```python
from build123d import *

# Parameters (mm, degrees)
BOSS_EXTRU_1_DEPTH       = 20
ESQUISSE2_W              = 10
ESQUISSE2_H              = 21
ENL_V_MAT_EXTRU_1_DEPTH  = 2.5
ESQUISSE3_R              = 1.5
ENL_V_MAT_EXTRU_2_DEPTH  = 20.384776311
ESQUISSE4_R              = 4.1
ENL_V_MAT_EXTRU_3_DEPTH  = 16.384776311
ESQUISSE5_R              = 1.25
ENL_V_MAT_EXTRU_4_DEPTH  = 17.207106781
BOSS_EXTRU_2_DEPTH       = 1
ENL_V_MAT_EXTRU_7_DEPTH  = 11
ENL_V_MAT_EXTRU_8_DEPTH  = 11
ESQUISSE11_R             = 1.5
ENL_V_MAT_EXTRU_9_DEPTH  = 12
ESQUISSE12_R             = 4.1
ENL_V_MAT_EXTRU_10_DEPTH = 7.5


with BuildPart() as part:
    # Esquisse1 → Boss.-Extru.1 (new body)
    with BuildSketch(Plane.XY):
        Polygon((0, 0), (0, 5), (-1, 5), (-1, 7.9), (0, 7.9), (0, 14.142135624), (11.313708499, 25.455844123), (18.384776311, 18.384776311), align=None)
    extrude(amount=BOSS_EXTRU_1_DEPTH)

    # Esquisse2 → Enlèv. mat.-Extru.1 (cut)
    with BuildSketch(Plane(origin=(0, 0, 0), x_dir=(0, 0, -1), z_dir=(0.707106781, -0.707106781, 0))):
        with Locations((-5, 15.5)):
            Rectangle(ESQUISSE2_W, ESQUISSE2_H)
    extrude(amount=-ENL_V_MAT_EXTRU_1_DEPTH, mode=Mode.SUBTRACT)

    # Esquisse3 → Enlèv. mat.-Extru.2 (cut, through all)
    with BuildSketch(Plane.ZY.offset(1)):
        with Locations((15, 6.45)):
            Circle(ESQUISSE3_R)
    extrude(amount=-ENL_V_MAT_EXTRU_2_DEPTH, mode=Mode.SUBTRACT)

    # Esquisse4 → Enlèv. mat.-Extru.3 (cut, through all)
    with BuildSketch(Plane.ZY.offset(-3)):
        with Locations((15, 6.45)):
            Circle(ESQUISSE4_R)
    extrude(amount=-ENL_V_MAT_EXTRU_3_DEPTH, mode=Mode.SUBTRACT)

    # Esquisse5 → Enlèv. mat.-Extru.4 (cut, through all)
    with BuildSketch(Plane(origin=(-1.767766953, 1.767766953, 0), x_dir=(0, 0, -1), z_dir=(0.707106781, -0.707106781, 0))):
        with Locations((-5, 11.5)):
            Circle(ESQUISSE5_R)
    extrude(amount=-ENL_V_MAT_EXTRU_4_DEPTH, mode=Mode.SUBTRACT)

    # Esquisse6 → Boss.-Extru.2 (add)
    with BuildSketch(Plane.XY.offset(20)):
        Polygon((0, 9.121677477), (13.823937572, 22.94561505), (15.874547238, 20.895005384), (0, 5.020458146), align=None)
    extrude(amount=BOSS_EXTRU_2_DEPTH)

    # Esquisse9 → Enlèv. mat.-Extru.7 (cut, through all)
    with BuildSketch(Plane(origin=(0, 0, 10), x_dir=(-1, 0, 0), z_dir=(0, 0, -1))):
        Polygon((-18.384776311, 18.384776311), (-12.02081528, 12.02081528), (-4.949747468, 19.091883092), (-11.313708499, 25.455844123), align=None)
    extrude(amount=ENL_V_MAT_EXTRU_7_DEPTH, mode=Mode.SUBTRACT)

    # Esquisse10 → Enlèv. mat.-Extru.8 (cut, through all)
    with BuildSketch(Plane(origin=(0, 0, 10), x_dir=(-1, 0, 0), z_dir=(0, 0, -1))):
        Polygon((-11.313708499, 25.455844123), (-4.242640687, 18.384776311), (-11.313708499, 11.313708499), (-18.384776311, 18.384776311), align=None)
    extrude(amount=ENL_V_MAT_EXTRU_8_DEPTH, mode=Mode.SUBTRACT)

    # Esquisse11 → Enlèv. mat.-Extru.9 (cut, through all)
    with BuildSketch(Plane(origin=(0, 0, 10), x_dir=(-1, 0, 0), z_dir=(0, 0, -1))):
        with Locations((-11.313708499, 18.384776311)):
            Circle(ESQUISSE11_R)
    extrude(amount=-ENL_V_MAT_EXTRU_9_DEPTH, mode=Mode.SUBTRACT)

    # Esquisse12 → Enlèv. mat.-Extru.10 (cut)
    with BuildSketch(Plane(origin=(0, 0, 10), x_dir=(-1, 0, 0), z_dir=(0, 0, -1))):
        with Locations((-11.313708499, 18.384776311)):
            Circle(ESQUISSE12_R)
    extrude(amount=-ENL_V_MAT_EXTRU_10_DEPTH, mode=Mode.SUBTRACT)


solid = part.part
```
Can you work these out from the model? Positions are in its coordinate system, mm. A direction names the side the tool comes from. Round coordinates to 2 decimals unless told otherwise and drop trailing zeros. Loops run counter-clockwise (first coordinate to the right, second up) from the corner with the lowest first, then second, coordinate; pieces in that order, holes last. Notation, with made-up numbers: (-26, 68) -> (-9, 68) arc R35 ccw to (-9, 103) -> close; hole circle Ø9 at (88.5, -2). An arc over 180 degrees is marked (long way). One line per item, written item: value. Start each with the question number.
1. If I drill on probe 1 along Z at (x, y) = (3.5, 12.75); probe 2 along X at (y, z) = (13.5, 6); probe 3 along X at (y, z) = (17, 13), over which ranges is the centre line in solid material (lowest first)?
2. If we section it at A-A, the plane z = 15: Write out the boundary of the cut face in (x, y).
3. If we section it at C-C, the plane z = 5.5: Write out the boundary of the cut face in (x, y).
4. If we mould it in two halves opening along Y, with no side actions, what happens to faces 1 (the flat face through (14.27, 19.29, 20.49)), 2 (the flat face through (0, 2, 10)), 3 (the flat face through (3, 8, 14))? For each: pulls with the +Y half, pulls with the -Y half, needs draft (parallel to the pull), parting line crosses it, or undercut.
5. If we section it at D-D, the plane z = 12.25: Write out the boundary of the cut face in (x, y), then the cut area to 3 significant figures.
6. For pin 1 (6 mm diameter, centred on x = 3.5, z = 7.5, fed in from -Y); pin 2 (5 mm diameter, centred on y = 6.45, z = 15, fed in from +X); pin 3 (4 mm diameter, centred on x = 11.5, y = 9.5, fed in from +Z); pin 4 (1.8 mm diameter, centred on x = 11.31, y = 18.38, fed in from -Z), each with a flat end and sliding along its axis, tell me the tip position at first contact or that it passes through.
7. For faces 4 (the flat face through (2.66, 4.41, 5.07)), 5 (the flat face through (-0.5, 7.9, 17.7)), 6 (the flat face through (11.4, 16.6, 17.5)), 7 (the flat face through (-0.5, 5, 17.7)), which set-ups out of +Z, -Z, +X, -X, +Y, -Y let a thin tool reach every point of the face, with its end or its side?
8. If we section it at B-B, the plane y = 6.45: Write out the boundary of the cut face in (x, z), then the cut area to 3 significant figures.
Calculated:
1. probe 1: z = 0 to 3.75, 6.25 to 20
1. probe 2: x = 0 to 1.7, 3.82 to 9.13
1. probe 3: x = 2.86 to 7.45, 15.17 to 17
2. outline: (0, 0) -> (3, 3) -> (3, 4.95) -> (0, 4.95) -> close; (0, 7.95) -> (3, 7.95) -> (3, 10.55) -> (10.55, 10.55) -> (18.38, 18.38) -> (11.31, 25.46) -> (0, 14.14) -> close; hole circle Ø8.2 at (11.31, 18.38)
3. outline: (-1, 5) -> (0, 5) -> (0, 0) -> (3.54, 3.54) -> (1.77, 5.3) -> (5.55, 9.09) -> (0.25, 14.39) -> (0, 14.14) -> (0, 7.9) -> (-1, 7.9) -> close; (1.87, 16.01) -> (7.17, 10.71) -> (9.55, 13.08) -> (4.24, 18.38) -> close
4. face 1: pulls with the -Y half
4. face 2: needs draft
4. face 3: undercut
5. outline: (-1, 5) -> (0, 5) -> (0, 0) -> (3.41, 3.41) -> (3, 3.41) -> (3, 9.49) -> (9.49, 9.49) -> (18.38, 18.38) -> (11.31, 25.46) -> (0, 14.14) -> (0, 7.9) -> (-1, 7.9) -> close; hole circle Ø8.2 at (11.31, 18.38)
5. area: 139 mm²
6. pin 1: stops at y = 0.5
6. pin 2: stops at x = 3
6. pin 3: stops at z = 20
6. pin 4: passes through
7. face 4: -Z, +X
7. face 5: +Z, -Z, -X, +Y
7. face 6: -Z
7. face 7: +Z, -Z, -X, -Y
8. outline: (-1, 0) -> (2.91, 0) -> (2.91, 10) -> (6.45, 10) -> (6.45, 10.9) -> (3, 10.9) -> (3, 13.5) -> (-1, 13.5) -> close; (-1, 16.5) -> (3, 16.5) -> (3, 19.1) -> (6.45, 19.1) -> (6.45, 20) -> (1.43, 20) -> (1.43, 21) -> (0, 21) -> (0, 20) -> (-1, 20) -> close
8. area: 74.8 mm²
